Input: part model. Units: mm. Frame: model coordinates. A direction names the side the tool comes from. Give positions to 0.01 mm unless a question says otherwise; leave off trailing zeros. Write each loop counter-clockwise with the first axis right and the second up, starting at its lowest first coordinate (ties: lowest second). Pieces come first, ordered by that corner, then holes. Notation, with made-up numbers: (54, 45) -> (83, 45) arc R22 ccw to (83, 72) -> close; hole circle Ø4 at (77.25, -17). An arc over 180 degrees is marked (long way). Return JSON: item names as keys, results as strings. Group by question number.
Item 1: Set-up query: faces 1 (the face through (0, -3, 6.1)), 2 (the face through (6, -14, 7.1)), 3 (the face through (0, -4, 0)), 4 (the face through (5.61, 18.57, -49.435)), 5 (the face through (2.1, 0.66, 4.99)). Return all of +Z, -Z, +X, -X, +Y, -Y with unobstructed straight access to the full face (end or side cutting, diameter ignored); none if empty.
Item 2: Mould query, pull axis Y, two halves, no side actions, for faces 6 (the face through (-3.202, -1.815, 2.021)), 7 (the face through (1.5, 17.3, 6.1)), 8 (the face through (9.139, 14.334, 6.593)). Classes: released by +Y, released by -Y, zero draft, split by the parting line, or undercut.
Item 3: Line query: line 1 (X direction, y = 0, z = -48); line 2 (Y direction, x = -16.5, z = -32.5); line 3 (Z direction, x = -13, y = 12). Output: solid intervals per line, ascending. Write a range as [from, to].
Item 4: Section D-D, the plane z = -21.5. Return loops of the section in (x, y).
Item 5: Section A-A, the plane x = 0. Return loops of the section in (y, z), then the cut area to 3 significant figures.
Item 6: Section B-B, the plane y = -12.5. Return loops of the section in (x, z), then the cut area to 3 significant figures.
Item 7: Section C-C, the plane x = -10. Return loops of the section in (y, z).
Item 8: Pin query (flat end, axial travel): P1, Ø2, axis at y = -14.5, z = -3.5, coming from the -X side; P2, Ø1.6, axis at y = 18, z = -58.5, coming from the -X side; P3, Ø10, axis at x = 5, z = -15.5, coming from the -Y side; P4, Ø2, axis at y = -13.5, z = -21, coming from the -X side. Return the tip coordinate at first contact, or that it passes through.
from build123d import *

# Parameters (mm, degrees)
SKETCH013_R     = 21.1
PAD004_DEPTH    = 4.1
SKETCH014_R     = 21.1
SKETCH014_R_2   = 2.2
PAD005_DEPTH    = 2
SKETCH012_R     = 17
SKETCH012_R_2   = 15
PAD006_DEPTH    = 1
CHAMFER003_SIZE = 0.2
SKETCH015_R     = 21.1
SKETCH015_R_2   = 18.1
PAD007_DEPTH    = 61.9
POCKET007_DEPTH = 15
CHAMFER004_SIZE = 5


with BuildPart() as part:
    # Sketch013 → Pad004 (new body)
    with BuildSketch(Plane.XY):
        Circle(SKETCH013_R)
        Polygon((2.125, -3.680608), (4.25, 0), (2.125, 3.680608), (-2.125, 3.680608), (-4.25, 0), (-2.125, -3.680608), align=None, mode=Mode.SUBTRACT)
    extrude(amount=PAD004_DEPTH)

    # Sketch014 → Pad005 (join)
    with BuildSketch(Plane.XY.offset(4.1)):
        Circle(SKETCH014_R)
        Circle(SKETCH014_R_2, mode=Mode.SUBTRACT)
    extrude(amount=PAD005_DEPTH)

    # Sketch012 → Pad006 (join)
    with BuildSketch(Plane.XY.offset(6.1)):
        Circle(SKETCH012_R)
        Circle(SKETCH012_R_2, mode=Mode.SUBTRACT)
    extrude(amount=PAD006_DEPTH)

    # Chamfer003
    chamfer003_edges = [part.edges().sort_by_distance(p)[0] for p in [
        (-2.2, 0, 6.1),
        (15, 0, 6.6),
    ]]
    chamfer(chamfer003_edges, length=CHAMFER003_SIZE)

    # Sketch015 → Pad007 (join)
    with BuildSketch(Plane.XY):
        Circle(SKETCH015_R)
        Circle(SKETCH015_R_2, mode=Mode.SUBTRACT)
    extrude(amount=-PAD007_DEPTH)

    # Sketch016 → Pocket007 (cut)
    with BuildSketch(Plane.XY.offset(-61.9)):
        with BuildLine():
            ThreePointArc((8.07462, 19.493858), (0, 21.1), (-8.07462, 19.493858))
            Line((-8.07462, 19.493858), (-8.07462, 16.19909))
            ThreePointArc((8.07462, 16.19909), (0, 18.1), (-8.07462, 16.19909))
            Line((8.07462, 19.493858), (8.07462, 16.19909))
        make_face()
    extrude(amount=POCKET007_DEPTH, mode=Mode.SUBTRACT)

    # Chamfer004
    chamfer004_edges = [part.edges().sort_by_distance(p)[0] for p in [
        (8.07462, 17.846474, -46.9),
        (-8.07462, 17.846474, -46.9),
    ]]
    chamfer(chamfer004_edges, length=CHAMFER004_SIZE)


solid = part.part
Answer below:
{
 "1": {"face 1": "+Z", "face 2": "+Z, +X, -X, +Y, -Y", "face 3": "-Z", "face 4": "-Z, +Y", "face 5": "+Z, -Z"},
 "2": {"face 6": "undercut", "face 7": "zero draft", "face 8": "split by the parting line"},
 "3": {"line 1": "x = [-21.1, -18.1], [18.1, 21.1]", "line 2": "y = [-13.15, -7.44], [7.44, 13.15]", "line 3": "z = [0, 6.1]"},
 "4": {"outline": "circle Ø42.2 at (0, 0); hole circle Ø36.2 at (0, 0)"},
 "5": {"outline": "(-21.1, -61.9) -> (-18.1, -61.9) -> (-18.1, 0) -> (-3.68, 0) -> (-3.68, 4.1) -> (-2.2, 4.1) -> (-2.2, 5.9) -> (-2.4, 6.1) -> (-15, 6.1) -> (-15, 7.1) -> (-17, 7.1) -> (-17, 6.1) -> (-21.1, 6.1) -> close; (2.2, 4.1) -> (3.68, 4.1) -> (3.68, 0) -> (18.1, 0) -> (18.1, -46.9) -> (21.1, -46.9) -> (21.1, 6.1) -> (17, 6.1) -> (17, 7.1) -> (15, 7.1) -> (15, 6.1) -> (2.4, 6.1) -> (2.2, 5.9) -> close", "area": "549 mm2"},
 "6": {"outline": "(-17, -61.9) -> (-13.09, -61.9) -> (-13.09, 0) -> (13.09, 0) -> (13.09, -61.9) -> (17, -61.9) -> (17, 6.1) -> (11.52, 6.1) -> (11.52, 7.1) -> (8.29, 7.1) -> (8.29, 6.1) -> (-8.29, 6.1) -> (-8.29, 7.1) -> (-11.52, 7.1) -> (-11.52, 6.1) -> (-17, 6.1) -> close", "area": "698 mm2"},
 "7": {"outline": "(-18.58, -61.9) -> (-15.09, -61.9) -> (-15.09, 0) -> (15.09, 0) -> (15.09, -61.9) -> (18.58, -61.9) -> (18.58, 6.1) -> (13.75, 6.1) -> (13.75, 7.1) -> (11.18, 7.1) -> (11.18, 6.1) -> (-11.18, 6.1) -> (-11.18, 7.1) -> (-13.75, 7.1) -> (-13.75, 6.1) -> (-18.58, 6.1) -> close"},
 "8": {"P1": "stops at x = -16.22", "P2": "stops at x = -12.22", "P3": "stops at y = -21.1", "P4": "stops at x = -17"}
}
